Here's the drawing with two shaded views (mm, measured from the low corner). I have some questions. Give positions to 0.01 mm unless a question says otherwise; leave off trailing zeros. Write each loop counter-clockwise with the first axis right and the second up, starting at its lowest first coordinate (ties: lowest second). Pieces come first, ordered by that corner, then holes. Notation, with made-up numbers: M 51,73 L 65,73 A13 ccw 65,83 Z; hole C 29.5,37.5 d2. An arc over 180 degrees is marked long. Answer as a JSON object with one key per item and string values. Group by question number.
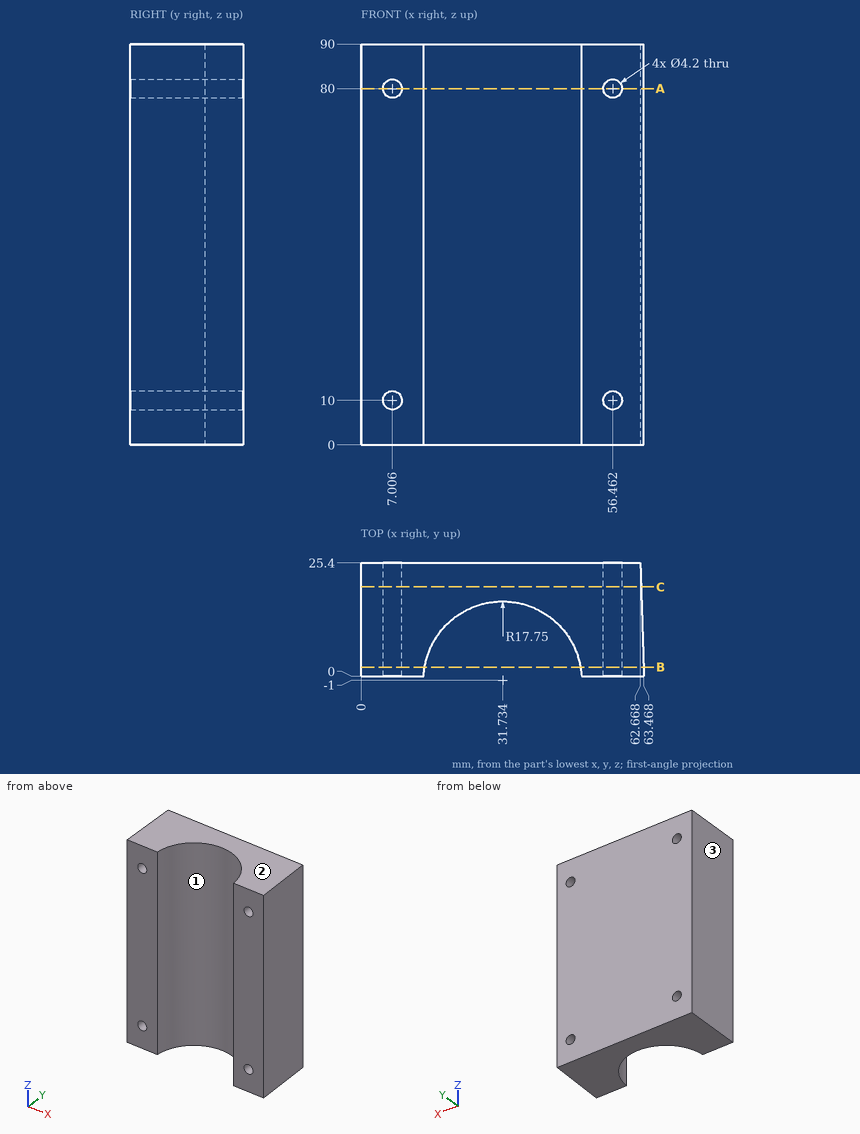
1) Please list where these lines run through material, in increasing order: line 1 along X through (y, z) = (9.5, 10) (1 decimal); line 2 along Z through (x, y) = (57, 11.75); line 3 along X through (y, z) = (13, 10) (1 decimal). Write a range as from..to.
2) If we section it at B-B, the plane y = 2: List the corners of the cut face in (x, z) for me (1 decimal), plus the area to 3 significant figures.
3) If we section it at C-C, the plane y = 20: List the corners of the cut face in (x, z) for me.
4) If we section it at A-A, the plane z = 80: Give the number of separate pieces and of enclosed holes in the cut face, plus the area to 3 significant figures.
5) We'd pull the mould along X, two halves only. Please class the marked faces 1, 2 and 3: released by +X, released by -X, zero draft, split by the parting line, or undercut.
6) I'm going to push a flat-ended pin straight in: pin 1 (8 mm diameter, centred on y = 13, z = 59.5, fed in from +X) (1 decimal). Where does the tip first touch, or does it pass through?
Taken from the geometry:
{
 "1": {"line 1": "0..4.9, 9.1..17.4, 46..54.4, 58.6..63.2", "line 2": "0..7.97, 12.03..77.97, 82.03..90", "line 3": "0..4.9, 9.1..20.8, 42.6..54.4, 58.6..63.1"},
 "2": {"outline": "M 0,0 L 14.2,0 L 14.2,90 L 0,90 Z; M 49.2,0 L 63.4,0 L 63.4,90 L 49.2,90 Z; hole C 7,10 d4.2; hole C 7,80 d4.2; hole C 56.5,10 d4.2; hole C 56.5,80 d4.2", "area": "2,500 mm²"},
 "3": {"outline": "M 0,0 L 62.84,0 L 62.84,90 L 0,90 Z; hole C 7.01,10 d4.2; hole C 7.01,80 d4.2; hole C 56.46,10 d4.2; hole C 56.46,80 d4.2"},
 "4": {"separate pieces": "3", "enclosed holes": "0", "area": "929 mm²"},
 "5": {"face 1": "undercut", "face 2": "zero draft", "face 3": "released by -X"},
 "6": {"pin 1": "x = 63.2"}
}
